Input: dimensioned drawing with shaded views. Units: mm. Origin: part minimum x, y, z. A direction names the side the tool comes from. Round coordinates to 2 decimals unless told otherwise and drop trailing zeros. Order: outer loops, then holes, each group sorted by start corner. A loop starts at its lowest first (then second) coordinate and runs counter-clockwise, first axis right, second up. Notation, with made-up numbers: M -29.75,38.25 L -12.75,38.25 A18 ccw -12.75,62.25 Z; hole C 56.5,34.5 d5. An arc over 180 degrees is marked long. Use CSV: the item, a comma, the result in double quotes. Start each with the question number.
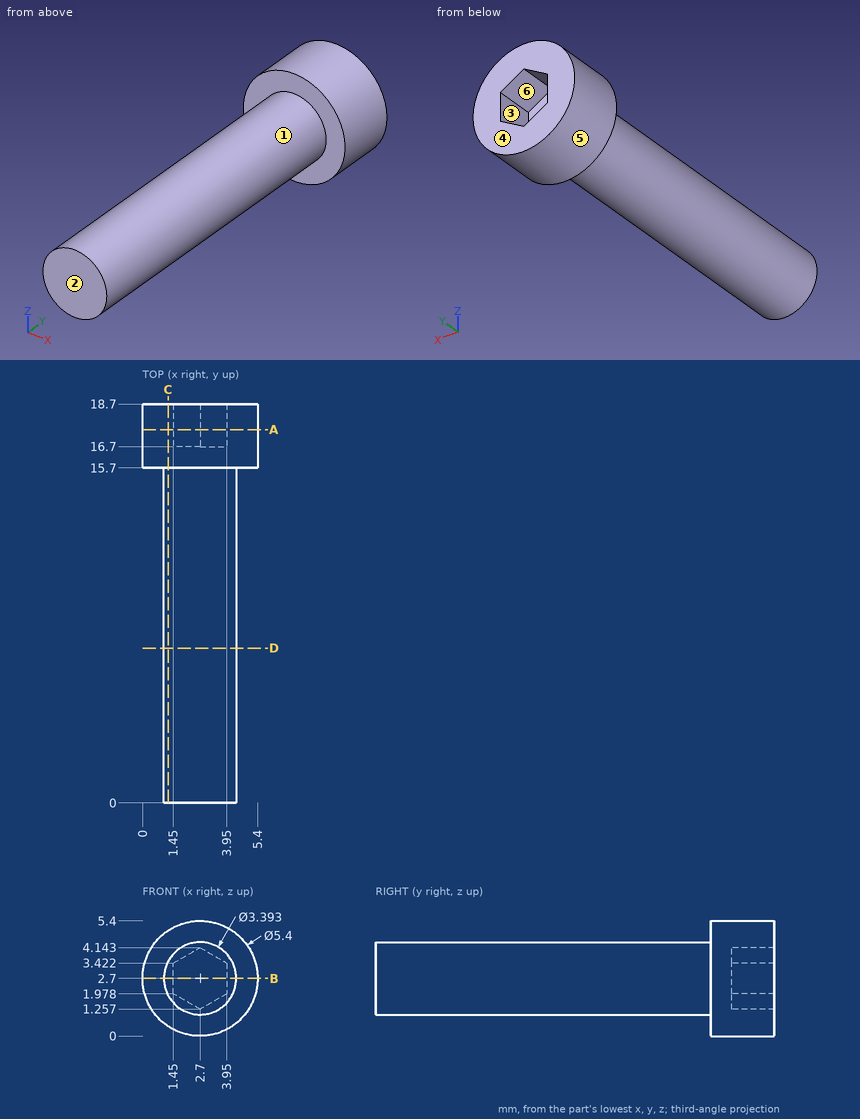
(1) Section B-B on z = 2.7. Return loops of the section in (x, y).
(2) Section A-A on y = 17.5. Return loops of the section in (x, z).
(3) Reachability of the marked faces 1 and 2 from +Z, -Z, +X, -X, +Y, -Y: full face, straight path, thin tool, end or side. Return the list, or none.
(4) Contact query for flat-ended pins moving along their axis: P1, Ø1.2, axis at x = 2.5, z = 2.5, coming from the +Y side; P2, Ø0.7, axis at y = 17.5, z = 2.5, coming from the +X side; P3, Ø1.5, axis at x = 2.5, y = 9.5, coming from the +Z side; P4, Ø2, axis at y = 11, z = 3, coming from the +X side. Output: stop coordinate, or through.
(5) Section C-C on x = 1.2. Return loops of the section in (y, z) (1 decimal).
(6) Section D-D on y = 7.25. Return loops of the section in (x, z).
(7) Line query: line 1 along Y through (x, z) = (5, 3); line 2 along Z through (x, y) = (1.55, 2.5) (1 decimal); line 3 along Z through (x, y) = (2.8, 10.75). Output: solid intervals per line, ascending.
(8) Draft query along X for the marked faces 3, 4, 5 and 6. Return one class per face: pulls with the +X half, pulls with the -X half, needs draft (parallel to the pull), parting line crosses it, or undercut.
Results below:
1,outline,"M 0,15.7 L 1,15.7 L 1,0 L 4.4,0 L 4.4,15.7 L 5.4,15.7 L 5.4,18.7 L 3.95,18.7 L 3.95,16.7 L 1.45,16.7 L 1.45,18.7 L 0,18.7 Z"
2,outline,"C 2.7,2.7 d5.4; hole M 1.45,1.98 L 2.7,1.26 L 3.95,1.98 L 3.95,3.42 L 2.7,4.14 L 1.45,3.42 Z"
3,face 1,"-Y"
3,face 2,"+Z, -Z, +X, -X, -Y"
4,P1,"stops at y = 16.7"
4,P2,"stops at x = 5.4"
4,P3,"stops at z = 4.4"
4,P4,"stops at x = 4.4"
5,outline,"M 0,1.9 L 15.7,1.9 L 15.7,0.5 L 18.7,0.5 L 18.7,4.9 L 15.7,4.9 L 15.7,3.5 L 0,3.5 Z"
6,outline,"C 2.7,2.7 d3.39"
7,line 1,"y = 15.7 to 18.7"
7,line 2,"z = 1.5 to 3.9"
7,line 3,"z = 1.01 to 4.39"
8,face 3,"undercut"
8,face 4,"needs draft"
8,face 5,"parting line crosses it"
8,face 6,"undercut"
